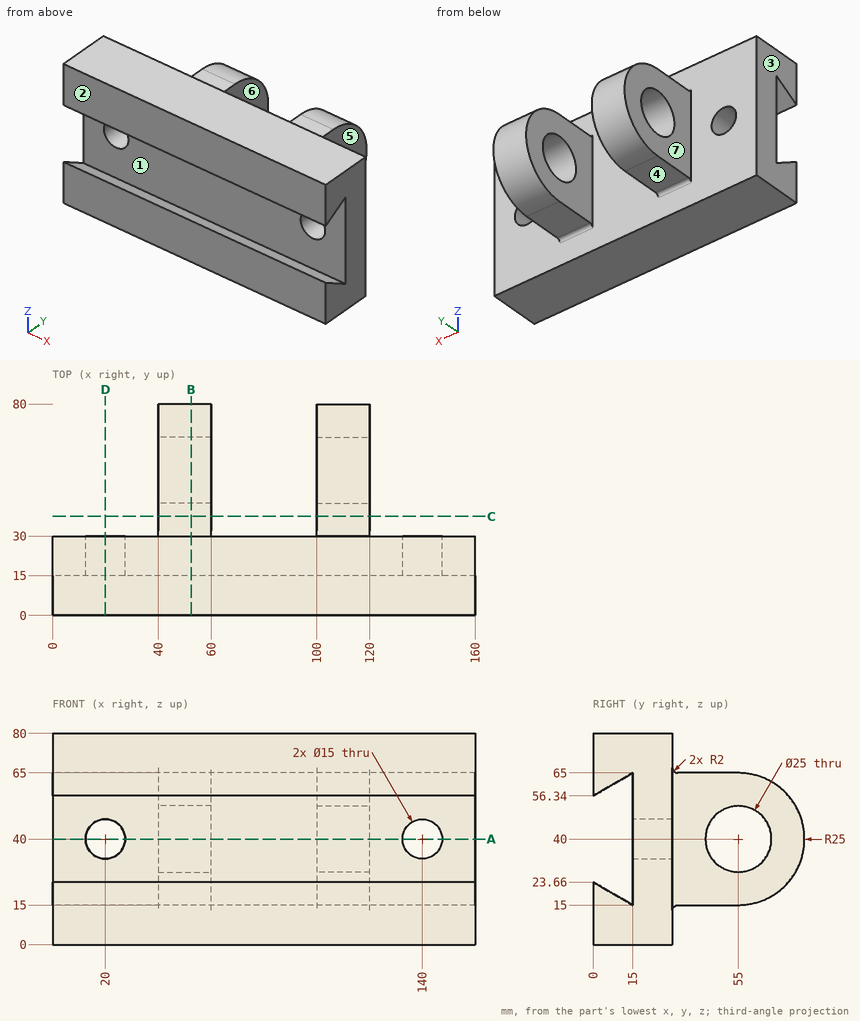
Drawing for the job (mm, zero at the part's lowest x, y, z). A direction names the side the tool comes from. Give positions to 0.01 mm unless a question says otherwise; leave off trailing zeros. Loops run counter-clockwise (first coordinate to the right, second up) from the corner with the lowest first, then second, coordinate; pieces in that order, holes last. Notation, with made-up numbers: M 57.5,-30.5 L 83.5,-30.5 A9 cw 83.5,-15.5 Z; hole C 29.5,61 d4. An arc over 180 degrees is marked long. One line per question, with ' | ' between items. Start each with the question number.
1. Saw through at D-D on x = 20. Give the cut face in (y, z).
2. Two-plate mould, pull along Y, no slides. Class the marked faces 1, 2 and 3: pulls with the +Y half, pulls with the -Y half, needs draft (parallel to the pull), parting line crosses it, or undercut.
3. Flat gauge pins, fed straight in: pin 1 (12 mm diameter, centred on x = 20, z = 40, fed in from -Y); pin 2 (15 mm diameter, centred on y = 47.5, z = 44.5, fed in from +X); pin 3 (15 mm diameter, centred on y = 60.5, z = 48, fed in from -X); pin 4 (6 mm diameter, centred on x = 112, y = 43.5, fed in from +Z). Where does each tip first touch, or does it go through?
4. 3-axis set-ups, long thin cutter, end or side, ignore diameter. For the marked faces 4, 5, 6 and 7: which of +Z, -Z, +X, -X, +Y, -Y reach the whole face in a straight line?
5. Probe L1, parallel to X at y = 20.5, z = 40; L2, parallel to Y at x = 53.5, z = 40; L3, parallel to Z at x = 20, y = 22. List the from-to ranges inside material, lowest first. Write a range as from..to.
6. Saw through at B-B on x = 52.5. Give the cut face in (y, z).
7. Saw through at A-A on z = 40. Give the cut face in (x, y), plus the area to 3 significant figures.
8. Saw through at C-C on y = 37.5. Give the cut face in (x, z).
Result sheet:
1) outline: M 0,0 L 30,0 L 30,32.5 L 15,32.5 L 15,15 L 0,23.66 Z; M 0,56.34 L 15,65 L 15,47.5 L 30,47.5 L 30,80 L 0,80 Z
2) face 1: undercut | face 2: pulls with the -Y half | face 3: needs draft
3) pin 1: passes through | pin 2: stops at x = 120 | pin 3: stops at x = 40 | pin 4: stops at z = 65
4) face 4: -Z, +X, -X, +Y | face 5: +Z, -Z, +X, +Y | face 6: +Z, -Z, +Y | face 7: +Z, -Z, -X, +Y
5) L1: x = 0..12.5, 27.5..132.5, 147.5..160 | L2: y = 15..42.5, 67.5..80 | L3: z = 0..32.5, 47.5..80
6) outline: M 0,0 L 30,0 L 30,13 A2 cw 32,15 L 55,15 A25 ccw 55,65 L 32,65 A2 cw 30,67 L 30,80 L 0,80 L 0,56.34 L 15,65 L 15,15 L 0,23.66 Z; hole C 55,40 d25
7) outline: M 0,15 L 12.5,15 L 12.5,30 L 0,30 Z; M 27.5,15 L 132.5,15 L 132.5,30 L 120,30 L 120,42.5 L 100,42.5 L 100,30 L 60,30 L 60,42.5 L 40,42.5 L 40,30 L 27.5,30 Z; M 40,67.5 L 60,67.5 L 60,80 L 40,80 Z; M 100,67.5 L 120,67.5 L 120,80 L 100,80 Z; M 147.5,15 L 160,15 L 160,30 L 147.5,30 Z | area: 2,950 mm^2
8) outline: M 40,15 L 60,15 L 60,65 L 40,65 Z; M 100,15 L 120,15 L 120,65 L 100,65 Z
